Part model, mm, in its own coordinate system. Face numbers are marked on the shaded views. A direction names the side the tool comes from. Coordinates: 2 decimals unless noted, no trailing zeros. Loops run counter-clockwise (first coordinate to the right, second up) from the corner with the lowest first, then second, coordinate; pieces in that order, holes last. Notation, with made-up numbers: (23.5, 27) -> (60.5, 27) arc R19 cw to (60.5, 35) -> close; hole circle Ø5 at (1.5, 5.5). An arc over 180 degrees is marked (long way). One line per question, with ' | ' between items. Start each with the question number.
1) Cut at A-A (y = 33.5). List the corners of the cut face in (x, z).
2) Probe L1, parallel to X at y = 8, z = -140 (3 decimals); L2, parallel to X at y = 15.5, z = 0; L3, parallel to Z at x = 1, y = 12. List the from-to ranges inside material, lowest first. Write a range as from..to.
3) Drop flat-ended pins along their axis: pin 1 (1.5 mm diameter, centred on x = -17, z = -71.5, fed in from -Y); pin 2 (12 mm diameter, centred on x = 9, y = 6, fed in from -Z); pin 3 (6 mm diameter, centred on y = 24.5, z = -25, fed in from -X); pin 4 (4 mm diameter, centred on x = 11.5, y = 25, fed in from +Z). Give the stop position or say it passes through.
4) 3-axis set-ups, long thin cutter, end or side, ignore diameter. For the marked faces 1 and 2: which of +Z, -Z, +X, -X, +Y, -Y reach the whole face in a straight line?
from build123d import *

# Parameters (mm, degrees)
BOSS_EXTRUDE1_DEPTH      = 20
SKETCH2_R                = 15.01
BOSS_EXTRUDE2_DEPTH      = 20
CHAMFER1_SIZE            = 1
SKETCH3_R                = 18.485
CUT_EXTRUDE1_DEPTH       = 20
CHAMFER3_SIZE            = 1
SKETCH5_R                = 2.65
CUT_EXTRUDE2_DEPTH       = 40
FILLET3_R                = 5
SKETCH6_R                = 3.65
CUT_EXTRUDE3_DEPTH       = 8
CHAMFER4_SIZE            = 0.5
BOSS_EXTRUDE3_DEPTH      = 6
BOSS_EXTRUDE3_DEPTH_BACK = 6
SKETCH7_R                = 18.485000000000003
SKETCH7_R_2              = 16.984999999999996


with BuildPart() as part:
    # Sketch1 → Boss-Extrude1 (new body)
    with BuildSketch(Plane(origin=(0, 0, 0), x_dir=(1, 0, 0), z_dir=(0, 1, 0))):
        with BuildLine():
            ThreePointArc((-23, 0), (1.41e-15, -22.999999999999982), (23, 0))
            ThreePointArc((23, 0), (17.845208734768505, 58.18386045047181), (20.033890701411753, 116.55459936267802))
            ThreePointArc((20.033890701411753, 116.55459936267802), (21.27316153822275, 124.05347023326534), (23.45051159720983, 131.33550314045155))
            ThreePointArc((23.45051159720983, 131.33550314045155), (-2.067e-14, 165.00000000000006), (-23.45051159720983, 131.3355031404515))
            ThreePointArc((-23.45051159720983, 131.3355031404515), (-21.27316153822273, 124.05347023326526), (-20.033890701411725, 116.55459936267786))
            ThreePointArc((-20.033890701411725, 116.55459936267786), (-17.845208734768505, 58.1838604504716), (-23, 0))
        make_face()
    extrude(amount=BOSS_EXTRUDE1_DEPTH)

    # Sketch2 → Boss-Extrude2 (add)
    with BuildSketch(Plane(origin=(0, 20, 0), x_dir=(1, 0, 0), z_dir=(0, 1, 0))):
        with Locations(Location((0, 0, 0), (0, 0, 90))):
            Circle(SKETCH2_R)
    extrude(amount=BOSS_EXTRUDE2_DEPTH)

    # Chamfer1
    chamfer1_edges = [part.edges().sort_by_distance(p)[0] for p in [
        (-2.76e-15, 40, 15.01),
    ]]
    chamfer(chamfer1_edges, length=CHAMFER1_SIZE)

    # Sketch3 → Cut-Extrude1 (cut)
    with BuildSketch(Plane(origin=(0, 20, 0), x_dir=(1, 0, 0), z_dir=(0, 1, 0))):
        with Locations(Location((0, 140.00000000000009, 0), (0, 0, 270))):
            Circle(SKETCH3_R)
    extrude(amount=-CUT_EXTRUDE1_DEPTH, mode=Mode.SUBTRACT)

    # Chamfer3
    # the kernel refuses this chamfer: 1 mm, written as the material it adds along each edge
    with BuildSketch(Plane(origin=(0, 20, 0), x_dir=(6e-17, 0, -1), z_dir=(1, 0, 6e-17))) as chamfer3_piece_1:
        Polygon((15.01, CHAMFER3_SIZE), (15.01 + CHAMFER3_SIZE, 0), (15.01, 0), align=None)
    revolve(axis=Axis((0, 20, 0), (0, 1, 0)))
    # the kernel refuses this chamfer: 1 mm, written as the material it takes off along each edge
    with BuildSketch(Plane(origin=(-79.73173943051358, 20, -110.54071067753486), x_dir=(0.9380204638883933, 0, -0.3465798743819428), z_dir=(-0.3465798743819428, 0, -0.9380204638883933))) as chamfer3_2_piece_1:
        Polygon((60.00000000000017 + CHAMFER3_SIZE, 0), (60.00000000000017, CHAMFER3_SIZE), (60.00000000000017, 0), align=None)
    revolve(axis=Axis((-79.73173943051358, 20, -110.54071067753486), (0, -1, 0)), revolution_arc=14.525766875036835, mode=Mode.SUBTRACT)
    with BuildSketch(Plane(origin=(-482.16572850262514, 20, -70.00000000000004), x_dir=(0.9949641454850282, 0, -0.1002314780857173), z_dir=(-0.1002314780857173, 0, -0.9949641454850282))) as chamfer3_2_piece_2:
        Polygon((464.4708454051196 + CHAMFER3_SIZE, 0), (464.4708454051196, CHAMFER3_SIZE), (464.4708454051196, 0), align=None)
    revolve(axis=Axis((-482.16572850262514, 20, -70.00000000000004), (0, -1, 0)), revolution_arc=14.737763084908373, mode=Mode.SUBTRACT)
    with BuildSketch(Plane(origin=(0, 20, -1.599e-14), x_dir=(-0.9937354343699007, 0, -0.11175816067592001), z_dir=(0.11175816067592001, 0, -0.9937354343699007))) as chamfer3_2_piece_3:
        Polygon((23.000000000000004 - CHAMFER3_SIZE, 0), (23.000000000000004, -CHAMFER3_SIZE), (23.000000000000004, 0), align=None)
    revolve(axis=Axis((0, 20, -1.599e-14), (0, 1, 0)), revolution_arc=192.83335153216495, mode=Mode.SUBTRACT)
    with BuildSketch(Plane(origin=(482.16572850261997, 20, -69.99999999999986), x_dir=(-0.9877285445231084, 0, 0.15618041597544133), z_dir=(0.15618041597544133, 0, 0.9877285445231084))) as chamfer3_2_piece_4:
        Polygon((464.4708454051149 + CHAMFER3_SIZE, 0), (464.47084540511446, CHAMFER3_SIZE), (464.4708454051149, 0), align=None)
    revolve(axis=Axis((482.16572850261997, 20, -69.99999999999986), (0, -1, 0)), revolution_arc=14.737763084908554, mode=Mode.SUBTRACT)
    with BuildSketch(Plane(origin=(0, 20, -140.00000000000009), x_dir=(-1.8e-16, 0, 1), z_dir=(-1, 0, -1.8e-16))) as chamfer3_2_piece_5:
        Polygon((18.485 + CHAMFER3_SIZE, 0), (18.485, -CHAMFER3_SIZE), (18.485, 0), align=None)
    revolve(axis=Axis((0, 20, -140.00000000000009), (0, 1, 0)), mode=Mode.SUBTRACT)
    with BuildSketch(Plane(origin=(79.7317394305139, 20, -110.54071067753493), x_dir=(-0.9949641454850281, 0, -0.10023147808571735), z_dir=(-0.10023147808571735, 0, 0.9949641454850281))) as chamfer3_2_piece_6:
        Polygon((60.000000000000455 + CHAMFER3_SIZE, 0), (60.000000000000455, CHAMFER3_SIZE), (60.000000000000455, 0), align=None)
    revolve(axis=Axis((79.7317394305139, 20, -110.54071067753493), (0, -1, 0)), revolution_arc=14.525766875036666, mode=Mode.SUBTRACT)
    with BuildSketch(Plane(origin=(9.77e-15, 20, -140.00000000000006), x_dir=(0.9380204638883942, 0, 0.3465798743819405), z_dir=(-0.3465798743819405, 0, 0.9380204638883942))) as chamfer3_2_piece_7:
        Polygon((24.999999999999982 - CHAMFER3_SIZE, 0), (24.999999999999982, -CHAMFER3_SIZE), (24.999999999999982, 0), align=None)
    revolve(axis=Axis((9.77e-15, 20, -140.00000000000006), (0, 1, 0)), revolution_arc=220.55653408148345, mode=Mode.SUBTRACT)

    # Sketch5 → Cut-Extrude2 (cut)
    with BuildSketch(Plane(origin=(0, 40, 0), x_dir=(1, 0, 0), z_dir=(0, 1, 0))):
        with Locations(Location((0, 0, 0), (0, 0, 270))):
            Circle(SKETCH5_R)
    extrude(amount=-CUT_EXTRUDE2_DEPTH, mode=Mode.SUBTRACT)

    # Fillet3
    # the kernel refuses this fillet: 5 mm, written as the material it takes off along each edge
    with BuildSketch(Plane(origin=(482.16572850261997, 0, -69.99999999999986), x_dir=(-0.9868985080370148, 0, 0.1613422909045059), z_dir=(0.1613422909045059, 0, 0.9868985080370148))) as fillet3_piece_1:
        with BuildLine():
            CenterArc((464.4708454051144 + FILLET3_R, -FILLET3_R), FILLET3_R, 89.99999999999935, 90.00000000000068)
            Line((464.4708454051144 + FILLET3_R, 8.9e-16), (464.4708454051144 + FILLET3_R, FILLET3_R * 0.02))
            Line((464.4708454051144 + FILLET3_R, FILLET3_R * 0.02), (464.4708454051144 - FILLET3_R * 0.02, FILLET3_R * 0.02))
            Line((464.4708454051144 - FILLET3_R * 0.02, FILLET3_R * 0.02), (464.4708454051144 - FILLET3_R * 0.02, -FILLET3_R))
            Line((464.4708454051144 - FILLET3_R * 0.02, -FILLET3_R), (464.4708454051144, -FILLET3_R))
        make_face()
    revolve(axis=Axis((482.16572850261997, 0, -69.99999999999986), (0, -1, 0)), revolution_arc=15.03731633345655, mode=Mode.SUBTRACT)
    with BuildSketch(Plane(origin=(0, 0, -1.599e-14), x_dir=(-0.9763879588864252, 0, -0.21602442857603077), z_dir=(0.21602442857603077, 0, -0.9763879588864252))) as fillet3_piece_2:
        with BuildLine():
            CenterArc((23 - FILLET3_R, FILLET3_R), FILLET3_R, 269.99999999999994, 90.00000000000006)
            Line((23 - FILLET3_R, -8.9e-16), (23 - FILLET3_R, -FILLET3_R * 0.02))
            Line((23 - FILLET3_R, -FILLET3_R * 0.02), (23 + FILLET3_R * 0.02, -FILLET3_R * 0.02))
            Line((23 + FILLET3_R * 0.02, -FILLET3_R * 0.02), (23 + FILLET3_R * 0.02, FILLET3_R))
            Line((23 + FILLET3_R * 0.02, FILLET3_R), (23.000000000000004, FILLET3_R))
        make_face()
    revolve(axis=Axis((0, 0, -1.599e-14), (0, 1, 0)), revolution_arc=204.95127041750123, mode=Mode.SUBTRACT)
    with BuildSketch(Plane(origin=(-482.16572850262514, 0, -70.00000000000004), x_dir=(0.9949641454850282, 0, -0.1002314780857173), z_dir=(-0.1002314780857173, 0, -0.9949641454850282))) as fillet3_piece_3:
        with BuildLine():
            CenterArc((464.4708454051196 + FILLET3_R, -FILLET3_R), FILLET3_R, 90, 90)
            Line((464.4708454051196 + FILLET3_R, 8.9e-16), (464.4708454051196 + FILLET3_R, FILLET3_R * 0.02))
            Line((464.4708454051196 + FILLET3_R, FILLET3_R * 0.02), (464.4708454051196 - FILLET3_R * 0.02, FILLET3_R * 0.02))
            Line((464.4708454051196 - FILLET3_R * 0.02, FILLET3_R * 0.02), (464.4708454051196 - FILLET3_R * 0.02, -FILLET3_R))
            Line((464.4708454051196 - FILLET3_R * 0.02, -FILLET3_R), (464.4708454051196, -FILLET3_R))
        make_face()
    revolve(axis=Axis((-482.16572850262514, 0, -70.00000000000004), (0, -1, 0)), revolution_arc=15.037316333456364, mode=Mode.SUBTRACT)
    with BuildSketch(Plane(origin=(-79.73173943051358, 0, -110.54071067753486), x_dir=(0.9380204638883933, 0, -0.3465798743819428), z_dir=(-0.3465798743819428, 0, -0.9380204638883933))) as fillet3_piece_4:
        with BuildLine():
            CenterArc((60.00000000000017 + FILLET3_R, -FILLET3_R), FILLET3_R, 90, 90)
            Line((60.00000000000017 + FILLET3_R, 8.9e-16), (60.00000000000017 + FILLET3_R, FILLET3_R * 0.02))
            Line((60.00000000000017 + FILLET3_R, FILLET3_R * 0.02), (60.00000000000017 - FILLET3_R * 0.02, FILLET3_R * 0.02))
            Line((60.00000000000017 - FILLET3_R * 0.02, FILLET3_R * 0.02), (60.00000000000017 - FILLET3_R * 0.02, -FILLET3_R))
            Line((60.00000000000017 - FILLET3_R * 0.02, -FILLET3_R), (60.00000000000018, -FILLET3_R))
        make_face()
    revolve(axis=Axis((-79.73173943051358, 0, -110.54071067753486), (0, -1, 0)), revolution_arc=14.525766875036835, mode=Mode.SUBTRACT)
    with BuildSketch(Plane(origin=(9.77e-15, 0, -140.00000000000006), x_dir=(0.9380204638883942, 0, 0.3465798743819405), z_dir=(-0.3465798743819405, 0, 0.9380204638883942))) as fillet3_piece_5:
        with BuildLine():
            CenterArc((24.999999999999982 - FILLET3_R, FILLET3_R), FILLET3_R, 270, 90)
            Line((24.999999999999982 - FILLET3_R, -8.9e-16), (24.999999999999982 - FILLET3_R, -FILLET3_R * 0.02))
            Line((24.999999999999982 - FILLET3_R, -FILLET3_R * 0.02), (24.999999999999982 + FILLET3_R * 0.02, -FILLET3_R * 0.02))
            Line((24.999999999999982 + FILLET3_R * 0.02, -FILLET3_R * 0.02), (24.999999999999982 + FILLET3_R * 0.02, FILLET3_R))
            Line((24.999999999999982 + FILLET3_R * 0.02, FILLET3_R), (24.999999999999986, FILLET3_R))
        make_face()
    revolve(axis=Axis((9.77e-15, 0, -140.00000000000006), (0, 1, 0)), revolution_arc=220.55653408148345, mode=Mode.SUBTRACT)
    with BuildSketch(Plane(origin=(79.7317394305139, 0, -110.54071067753493), x_dir=(-0.9949641454850281, 0, -0.10023147808571735), z_dir=(-0.10023147808571735, 0, 0.9949641454850281))) as fillet3_piece_6:
        with BuildLine():
            CenterArc((60.000000000000455 + FILLET3_R, -FILLET3_R), FILLET3_R, 90, 90)
            Line((60.000000000000455 + FILLET3_R, 8.9e-16), (60.000000000000455 + FILLET3_R, FILLET3_R * 0.02))
            Line((60.000000000000455 + FILLET3_R, FILLET3_R * 0.02), (60.000000000000455 - FILLET3_R * 0.02, FILLET3_R * 0.02))
            Line((60.000000000000455 - FILLET3_R * 0.02, FILLET3_R * 0.02), (60.000000000000455 - FILLET3_R * 0.02, -FILLET3_R))
            Line((60.000000000000455 - FILLET3_R * 0.02, -FILLET3_R), (60.000000000000455, -FILLET3_R))
        make_face()
    revolve(axis=Axis((79.7317394305139, 0, -110.54071067753493), (0, -1, 0)), revolution_arc=14.525766875036666, mode=Mode.SUBTRACT)

    # Sketch6 → Cut-Extrude3 (cut)
    with BuildSketch(Plane.XZ):
        with Locations(Location((0, 0, 0), (0, 0, 270))):
            Circle(SKETCH6_R)
    extrude(amount=-CUT_EXTRUDE3_DEPTH, mode=Mode.SUBTRACT)

    # Chamfer4
    chamfer4_edges = [part.edges().sort_by_distance(p)[0] for p in [
        (1.12e-15, 0, 3.65),
    ]]
    chamfer(chamfer4_edges, length=CHAMFER4_SIZE)

    # Sketch7 → Boss-Extrude3 (add, two sides: drawn at the far end of the back side and taken through both)
    with BuildSketch(Plane(origin=(0, 10, 0), x_dir=(1, 0, 0), z_dir=(0, 1, 0)).offset(-BOSS_EXTRUDE3_DEPTH_BACK)):
        with Locations(Location((0, 140.00000000000009, 0), (0, 0, 270))):
            Circle(SKETCH7_R)
        with Locations(Location((0, 140.00000000000009, 0), (0, 0, 270))):
            Circle(SKETCH7_R_2, mode=Mode.SUBTRACT)
    extrude(amount=BOSS_EXTRUDE3_DEPTH + BOSS_EXTRUDE3_DEPTH_BACK)


solid = part.part
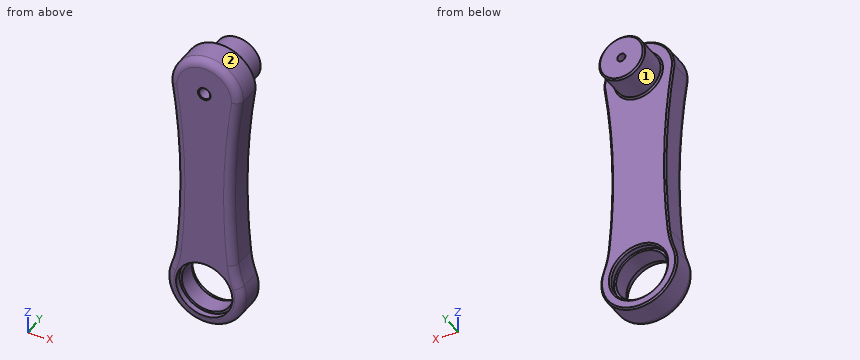
Reported:
1) outline: circle Ø30.02 at (0, 0); hole circle Ø5.3 at (0, 0)
2) L1: x = -25..-16.985, 16.985..25 | L2: x = -23..-2.65, 2.65..23 | L3: z = -164.98..-156.96, -123.04..-2.45, 2.45..22.98
3) pin 1: stops at y = 1.48 | pin 2: stops at z = -164.82 | pin 3: passes through | pin 4: stops at z = 11.62
4) face 1: +Y | face 2: +Z, +Y, -Y
